Model file for the job. Use its own axes, mm. Coordinates: 2 decimals unless noted, no trailing zeros. Order: outer loops, then holes, each group sorted by start corner. A loop starts at its lowest first (then second) coordinate and runs counter-clockwise, first axis right, second up. Notation, with made-up numbers: (23, 17.5) -> (31, 17.5) arc R20 ccw to (31, 27.5) -> close; hole circle Ø4 at (-15.5, 63). An arc over 180 degrees is marked (long way). Write item = value, one per line. Start each with the question number.
Q1. Cut at A-A, the plane x = -14.5. List the corners of the cut face in (y, z).
Q2. Flat gauge pins, fed straight in: pin 1 (1.5 mm diameter, centred on y = 1, z = -94, fed in from +X); pin 2 (5.5 mm diameter, centred on x = -46.5, z = -83, fed in from +Y); pin 3 (1.5 mm diameter, centred on x = -15.5, y = 2, fed in from -Z). Where does each tip first touch, or does it go through?
Q3. Cut at B-B, the plane y = 1.6. Give the number of separate pieces and of enclosed holes in the cut face, plus the area to 3 significant figures.
Q4. Wall check: line 1 (X direction, y = 2.95, z = 20); line 2 (X direction, y = 1.35, z = 50); line 3 (X direction, y = 1.65, z = -20). Give the ranges that are in metal, low to high. Write a range as from..to.
from build123d import *

# Parameters (mm, degrees)
SKETCH2_W           = 135
SKETCH2_H           = 190
BOSS_EXTRUDE2_DEPTH = 3
SKETCH3_R           = 1.75
CUT_EXTRUDE1_DEPTH  = 117.577227622
FILLET1_SIZE        = 12.5
FILLET1_SIZE_2      = 50
FILLET2_SIZE        = 12.5
FILLET2_SIZE_2      = 50
CHAMFER2_SIZE       = 25
CHAMFER3_SIZE       = 25
CUT_EXTRUDE5_DEPTH  = 117.577227764
SKETCH8_R           = 1.75
CUT_EXTRUDE6_DEPTH  = 117.577227764
SKETCH9_R           = 1.75
CUT_EXTRUDE7_DEPTH  = 117.577227764
SKETCH11_R          = 1.75
CUT_EXTRUDE8_DEPTH  = 117.577227764
SKETCH12_W          = 16
SKETCH12_H          = 15
CUT_EXTRUDE9_DEPTH  = 117.577227764


with BuildPart() as part:
    # Sketch2 → Boss-Extrude2 (new body)
    with BuildSketch(Plane(origin=(0, 0, 0), x_dir=(1, 0, 0), z_dir=(0, 1, 0))):
        Rectangle(SKETCH2_W, SKETCH2_H)
    extrude(amount=BOSS_EXTRUDE2_DEPTH)

    # Sketch3 → Cut-Extrude1 (cut, through all)
    with BuildSketch(Plane(origin=(0, 3, 0), x_dir=(1, 0, 0), z_dir=(0, 1, 0))):
        with Locations(Location((-27.5, -50, 0), (0, 0, 270))):
            Circle(SKETCH3_R)
        with Locations(Location((27.5, -50, 0), (0, 0, 90))):
            Circle(SKETCH3_R)
        with Locations(Location((-50, -85, 0), (0, 0, 270))):
            Circle(SKETCH3_R)
        with Locations(Location((50, -85, 0), (0, 0, 90))):
            Circle(SKETCH3_R)
    extrude(amount=-CUT_EXTRUDE1_DEPTH, mode=Mode.SUBTRACT)

    # Fillet1
    # an asymmetric fillet: 50, 12.5 mm, written as the material it takes off along each edge
    with BuildSketch(Plane(origin=(-67.5, -125, 95), x_dir=(0, 0, -1), z_dir=(0, 1, 0))) as fillet1_piece_1:
        with BuildLine():
            Bezier((FILLET1_SIZE, 0), (0, 0), (0, -FILLET1_SIZE_2), weights=[1, 0.707106781, 1])
            Line((0, -FILLET1_SIZE_2), (0, 0))
            Line((0, 0), (FILLET1_SIZE, 0))
        make_face()
    extrude(amount=253, mode=Mode.SUBTRACT)

    # Fillet2
    # an asymmetric fillet: 50, 12.5 mm, written as the material it takes off along each edge
    with BuildSketch(Plane(origin=(67.5, -125, 95), x_dir=(0, 0, -1), z_dir=(0, 1, 0))) as fillet2_piece_1:
        with BuildLine():
            Bezier((FILLET2_SIZE, 0), (0, 0), (0, FILLET2_SIZE_2), weights=[1, 0.707106781, 1])
            Line((0, FILLET2_SIZE_2), (0, 0))
            Line((0, 0), (FILLET2_SIZE, 0))
        make_face()
    extrude(amount=253, mode=Mode.SUBTRACT)

    # Chamfer2
    chamfer2_edges = [part.edges().sort_by_distance(p)[0] for p in [
        (67.5, 1.5, -95),
    ]]
    chamfer(chamfer2_edges, length=CHAMFER2_SIZE)

    # Chamfer3
    chamfer3_edges = [part.edges().sort_by_distance(p)[0] for p in [
        (-67.5, 1.5, -95),
    ]]
    chamfer(chamfer3_edges, length=CHAMFER3_SIZE)

    # Sketch7 → Cut-Extrude5 (cut, through all)
    with BuildSketch(Plane(origin=(0, 3, 0), x_dir=(1, 0, 0), z_dir=(0, 1, 0))):
        with BuildLine():
            Line((24, 91.5), (24, 95))
            Line((24, 95), (-24, 95))
            Line((-24, 95), (-24, 91.5))
            ThreePointArc((-24, 91.5), (0, 67.5), (24, 91.5))
        make_face()
    extrude(amount=-CUT_EXTRUDE5_DEPTH, mode=Mode.SUBTRACT)

    # Sketch8 → Cut-Extrude6 (cut, through all)
    with BuildSketch(Plane(origin=(0, 3, 0), x_dir=(1, 0, 0), z_dir=(0, 1, 0))):
        with Locations(Location((-27, 91.5, 0), (0, 0, 270))):
            Circle(SKETCH8_R)
        with Locations(Location((27, 91.5, 0), (0, 0, 270))):
            Circle(SKETCH8_R)
    extrude(amount=-CUT_EXTRUDE6_DEPTH, mode=Mode.SUBTRACT)

    # Sketch9 → Cut-Extrude7 (cut, through all)
    with BuildSketch(Plane(origin=(0, 3, 0), x_dir=(1, 0, 0), z_dir=(0, 1, 0))):
        with Locations(Location((-56.25, -15, 0), (0, 0, 270))):
            Circle(SKETCH9_R)
        with Locations(Location((-35, 56.25, 0), (0, 0, 270))):
            Circle(SKETCH9_R)
        with Locations(Location((-56.25, 20, 0), (0, 0, 270))):
            Circle(SKETCH9_R)
        with Locations(Location((35, 56.25, 0), (0, 0, 270))):
            Circle(SKETCH9_R)
    extrude(amount=-CUT_EXTRUDE7_DEPTH, mode=Mode.SUBTRACT)

    # Sketch11 → Cut-Extrude8 (cut, through all)
    with BuildSketch(Plane(origin=(0, 3, 0), x_dir=(1, 0, 0), z_dir=(0, 1, 0))):
        with Locations(Location((62.5, 70, 0), (0, 0, 270))):
            Circle(SKETCH11_R)
        with Locations(Location((-46.5, 83, 0), (0, 0, 270))):
            Circle(SKETCH11_R)
    extrude(amount=-CUT_EXTRUDE8_DEPTH, mode=Mode.SUBTRACT)

    # Sketch12 → Cut-Extrude9 (cut, through all)
    with BuildSketch(Plane(origin=(0, 3, 0), x_dir=(1, 0, 0), z_dir=(0, 1, 0))):
        with Locations((-17.534965815, -16.5)):
            Rectangle(SKETCH12_W, SKETCH12_H)
        with Locations((10.465034185, -16.5)):
            Rectangle(SKETCH12_W, SKETCH12_H)
    extrude(amount=-CUT_EXTRUDE9_DEPTH, mode=Mode.SUBTRACT)


solid = part.part
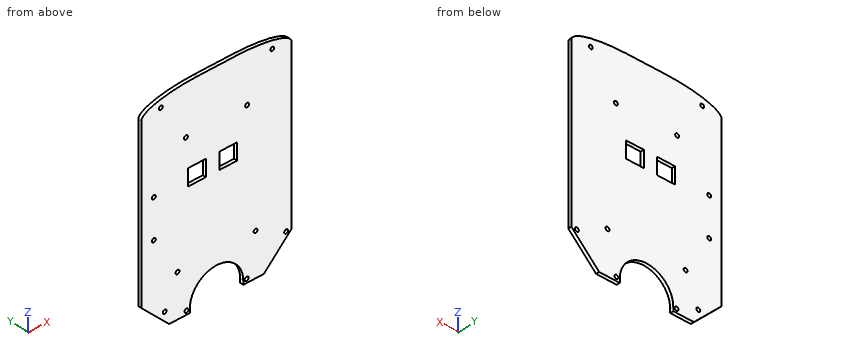
Here are the results:
q1.outline = (0, -72.38) -> (3, -72.38) -> (3, 9) -> (0, 9) -> close; (0, 24) -> (3, 24) -> (3, 95) -> (0, 95) -> close
q2.pin_1 = 44.25
q2.pin_2 = 3
q2.pin_3 = -73.84
q3.separate_pieces = 1
q3.enclosed_holes = 14
q3.area = 23,100 mm²
q4.line_1 = -67.5..-25.53, -9.53..2.47, 18.47..67.5
q4.line_2 = -67.5..-29.25, -25.75..25.75, 29.25..67.5
q4.line_3 = -67.5..-58, -54.5..67.5
